Source: three-view drawing plus pictorial views. Frame: mm from the lowest corner of the part. Round coordinates to 2 decimals unless told otherwise and drop trailing zeros. Loops run counter-clockwise (first coordinate to the right, second up) from the corner with the lowest first, then second, coordinate; pieces in that order, holes last. Notation, with made-up numbers: (-11.5, 89) -> (46.5, 89) arc R14 cw to (46.5, 104) -> close; hole circle Ø10 at (52, 78.25). An arc over 180 degrees is marked (long way). Put each result on its own line as item: value. Start each with the question number.
1. Cut plane C-C (x = 100.5). Return the cut outline in (y, z).
2. Material intervals for L1, parallel to X at y = 6.25, z = 4; L2, parallel to Z at x = 95.5, y = 5.25; L3, parallel to Y at x = 82, z = 11, sorted ascending.
3. Contact query for a flat-ended pin moving along its axis: pin 1 (1 mm diameter, centred on y = 6, z = 13.5, fed in from -X). Output: stop coordinate, or through.
4. Draft query along X for the marked faces 1 and 2. Return one class per face: pulls with the +X half, pulls with the -X half, needs draft (parallel to the pull), parting line crosses it, or undercut.
5. Cut plane A-A (y = 5.5). Return the cut outline in (x, z).
6. Cut plane B-B (z = 4.75). Return the cut outline in (x, y), then the cut area to 3 significant figures.
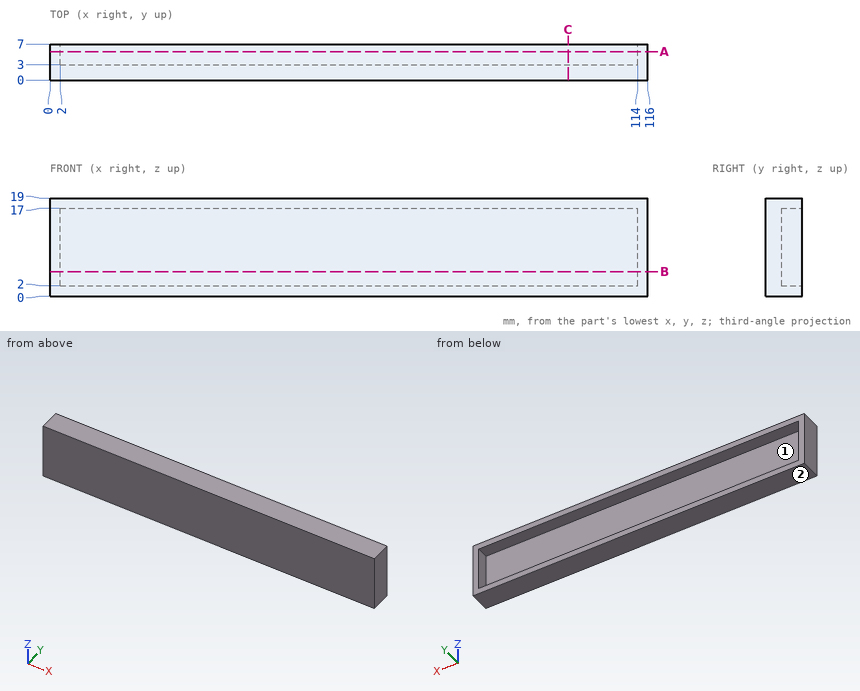
Solution:
1. outline: (0, 0) -> (7, 0) -> (7, 2) -> (3, 2) -> (3, 17) -> (7, 17) -> (7, 19) -> (0, 19) -> close
2. L1: x = 0 to 2, 114 to 116
2. L2: z = 0 to 2, 17 to 19
2. L3: y = 0 to 3
3. pin 1: stops at x = 0
4. face 1: undercut
4. face 2: needs draft
5. outline: (0, 0) -> (116, 0) -> (116, 19) -> (0, 19) -> close; hole (2, 2) -> (114, 2) -> (114, 17) -> (2, 17) -> close
6. outline: (0, 0) -> (116, 0) -> (116, 7) -> (114, 7) -> (114, 3) -> (2, 3) -> (2, 7) -> (0, 7) -> close
6. area: 364 mm^2
